```python
from build123d import *

# Parameters (mm, degrees)
F1_DEPTH = 76.2
F2_W     = 25.4
F2_H     = 25.4
F3_DEPTH = 12.7
F4_R     = 12.7
F5_DEPTH = 12.7
F7_D     = 25.4


with BuildPart() as f1:
    # F0 (on Front) → F1 (new body)
    with BuildSketch(Plane.XZ):
        Polygon((-70.789909, 90.538534), (-70.789909, 14.338534), (5.410091, 14.338534), (5.410091, 90.538534), (-11.810248, 90.538534), (-32.689909, 90.538534), align=None)
    extrude(amount=F1_DEPTH)

    # F2 (on face) → F3 (join)
    with BuildSketch(Plane.XZ.offset(76.2)):
        with Locations((-32.689909, 52.438534)):
            Rectangle(F2_W, F2_H)
    extrude(amount=F3_DEPTH)

    # F4 (on face) → F5 (join)
    with BuildSketch(Plane.YZ.offset(5.410091)):
        with Locations((-38.1, 51.235449)):
            Circle(F4_R)
    extrude(amount=F5_DEPTH)

    # F7 (through all)
    with Locations(Plane.XY.offset(90.538534)):
        with Locations((-32.689909, -38.1)):
            Hole(F7_D / 2)


solid = f1.part
```
The listing builds one solid part. Answer for the finished solid, in the listing's coordinates (mm). A direction names the side the tool comes from. Give positions to 0.01 mm unless a question says otherwise; leave off trailing zeros. Order: outer loops, then holes, each group sorted by start corner. A loop starts at its lowest first (then second) coordinate and runs counter-clockwise, first axis right, second up.
1) Find section D-D on x = -56.5. Write down the section's boundary in (y, z), then the cut area to 3 significant figures.
Reported:
outline: (-76.2, 14.34) - (0, 14.34) - (0, 90.54) - (-76.2, 90.54) - close
area: 5,810 mm2
2) For faces 4 (the face through (-45.39, -82, 52)), 5 (the face through (-33, -82, 65.139)), 6 (the face through (-33, -82, 39.739)), 7 (the face through (5.41, -38, 69)), determine the directions among +Z, -Z, +X, -X, +Y, -Y from which every point of the face is accessible in a straight line to the end or side of a thin tool.
Reported:
face 4: +Z, -Z, -X, -Y
face 5: +Z, +X, -X, -Y
face 6: -Z, +X, -X, -Y
face 7: +X
3) Find section B-B on x = -33. Write down the section's boundary in (y, z).
Reported:
outline: (-88.9, 39.74) - (-76.2, 39.74) - (-76.2, 14.34) - (-50.8, 14.34) - (-50.8, 90.54) - (-76.2, 90.54) - (-76.2, 65.14) - (-88.9, 65.14) - close; (-25.4, 14.34) - (0, 14.34) - (0, 90.54) - (-25.4, 90.54) - close
4) Find section A-A on y = -38.1. Write down the section's boundary in (x, z).
Reported:
outline: (-70.79, 14.34) - (-45.39, 14.34) - (-45.39, 90.54) - (-70.79, 90.54) - close; (-19.99, 14.34) - (5.41, 14.34) - (5.41, 38.54) - (18.11, 38.54) - (18.11, 63.94) - (5.41, 63.94) - (5.41, 90.54) - (-19.99, 90.54) - close
5) Consider line 1 along Y through (x, z) = (-11.5, 72); line 2 along X through (y, z) = (-61, 38.5); line 3 along Y through (x, z) = (-26.5, 68). Determine where each line is inside the solid, lowest interval first.
Reported:
line 1: y = -76.2 to 0
line 2: x = -70.79 to 5.41
line 3: y = -76.2 to -49.19, -27.01 to 0
6) Determine the mould class of faces 1 (the face through (11.67, -47.46, 59.82)), 2 (the face through (-15, -38, 90.539)), 3 (the face through (-22.612, -45.828, 51.905)) for opening direction Y: pulls with the +Y half, pulls with the -Y half, needs draft (parallel to the pull), parting line crosses it, or undercut.
Reported:
face 1: parting line crosses it
face 2: needs draft
face 3: undercut
7) Given P1, Ø1, axis at x = -8, z = 70, coming from the -Y side; P2, Ø10, axis at x = -30.5, y = -81.5, coming from the -Z side; P3, Ø1, axis at y = -56.5, z = 39, coming from the +X side; P4, Ø15, axis at x = -32.69, y = -38.1, coming from the -Z side, each flat-ended and moving along its own axis, determine where each tip first touches the part or whether it passes through.
Reported:
P1: stops at y = -76.2
P2: stops at z = 39.74
P3: stops at x = 5.41
P4: passes through
8) Find section C-C on z = 77.5. Write down the section's boundary in (x, y).
Reported:
outline: (-70.79, -76.2) - (5.41, -76.2) - (5.41, 0) - (-70.79, 0) - close; hole circle Ø25.4 at (-32.69, -38.1)
